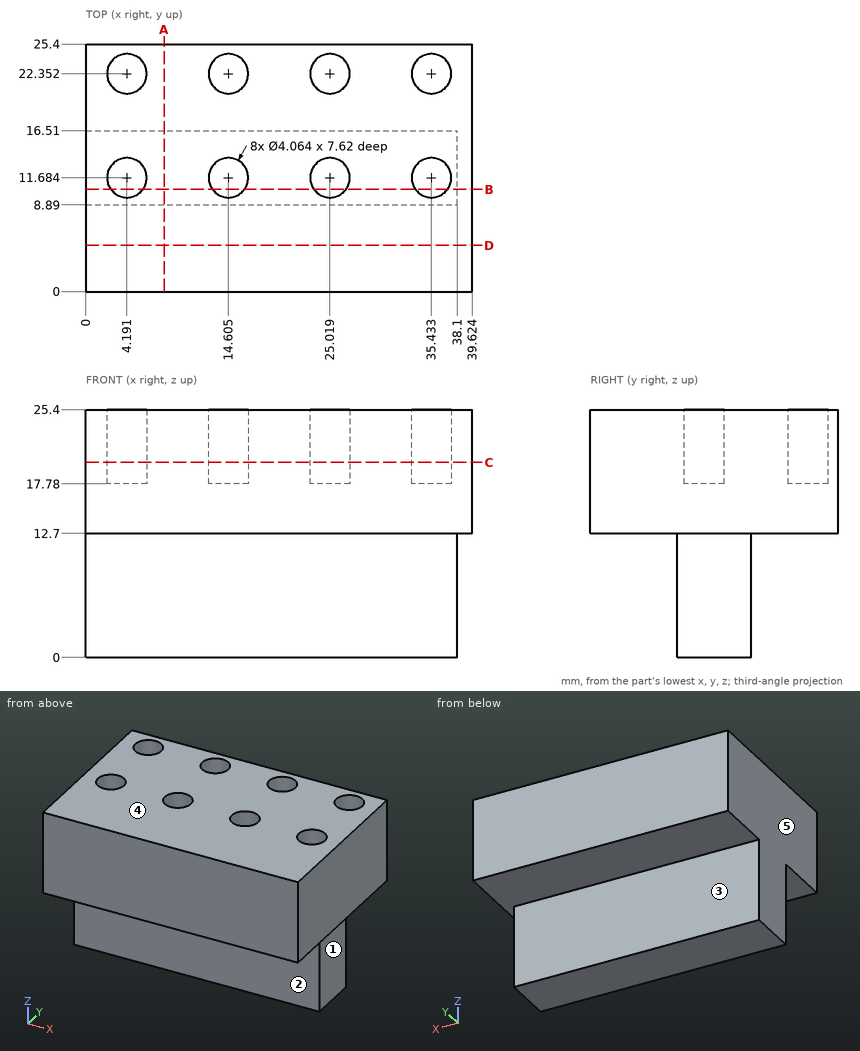
Answer from the drawing. Dimensions are ordinates in mm from the lowest x, y and z of the part. A direction names the side the tool comes from. Coordinates: 2 decimals unless noted, no trailing zeros. Write each loop counter-clockwise with the first axis right and the second up, starting at its lowest first coordinate (ties: lowest second). Pieces come first, ordered by that corner, then holes. Notation, with made-up numbers: (-17.5, 85) - (31.5, 85) arc R34 ccw to (31.5, 115) - close; hole circle Ø1 at (56, 7). An arc over 180 degrees is marked (long way). Answer as CSV lines item,"result".
1. Find section D-D (y = 4.75). Give the vertices of the cut face in (x, z), plus the area to 3 significant figures.
Computed values:
outline,"(0, 12.7) - (39.62, 12.7) - (39.62, 25.4) - (0, 25.4) - close"
area,"503 mm²"
2. A tool of negligible diameter and unlimited length cuts with its end or side. For the marked faces 1, 2, 3, 4 and 5, from which of +Z, -Z, +X, -X, +Y, -Y can it reach the whole face along a straight path? Write none if from no direction.
Computed values:
face 1,"-Z, +X, +Y, -Y"
face 2,"-Z, +X, -X, -Y"
face 3,"-Z, +X, -X, +Y"
face 4,"+Z, +X, -X, +Y, -Y"
face 5,"+Z, -Z, -X, +Y, -Y"
3. Find section C-C (z = 20). Give the number of separate pieces and of enclosed holes in the cut face, plus the area to 3 significant figures.
Computed values:
separate pieces,"1"
enclosed holes,"8"
area,"903 mm²"
4. Find section B-B (y = 10.5). Give the vertices of the cut face in (x, z), plus the area to 3 significant figures.
Computed values:
outline,"(0, 0) - (38.1, 0) - (38.1, 12.7) - (39.62, 12.7) - (39.62, 25.4) - (37.08, 25.4) - (37.08, 17.78) - (33.78, 17.78) - (33.78, 25.4) - (26.67, 25.4) - (26.67, 17.78) - (23.37, 17.78) - (23.37, 25.4) - (16.26, 25.4) - (16.26, 17.78) - (12.95, 17.78) - (12.95, 25.4) - (5.84, 25.4) - (5.84, 17.78) - (2.54, 17.78) - (2.54, 25.4) - (0, 25.4) - close"
area,"886 mm²"
5. Given P1, Ø1.2, axis at x = 4.5, y = 21.5, coming from the +Z side; P2, Ø8.5, axis at y = 13.5, z = 8, coming from the +X side; P3, Ø8, axis at x = 25, z = 4.5, coming from the -Y side, each flat-ended and moving along its own axis, determine where each tip first touches the part or whether it passes through.
Computed values:
P1,"stops at z = 17.78"
P2,"stops at x = 38.1"
P3,"stops at y = 8.89"
6. Find section A-A (x = 8). Give the vertices of the cut face in (y, z), plus the area to 3 significant figures.
Computed values:
outline,"(0, 12.7) - (8.89, 12.7) - (8.89, 0) - (16.51, 0) - (16.51, 12.7) - (25.4, 12.7) - (25.4, 25.4) - (0, 25.4) - close"
area,"419 mm²"
7. Straight lines are drawn through the part: line 1 (X direction, y = 22.5, z = 19.5); line 2 (Y direction, x = 10.5, z = 12.25); line 3 (X direction, y = 9, z = 9.5). For each, find the intervals that lie inside material, in ascending order. Write a range as [from, to].
Computed values:
line 1,"x = [0, 2.16], [6.22, 12.58], [16.63, 22.99], [27.05, 33.41], [37.46, 39.62]"
line 2,"y = [8.89, 16.51]"
line 3,"x = [0, 38.1]"
